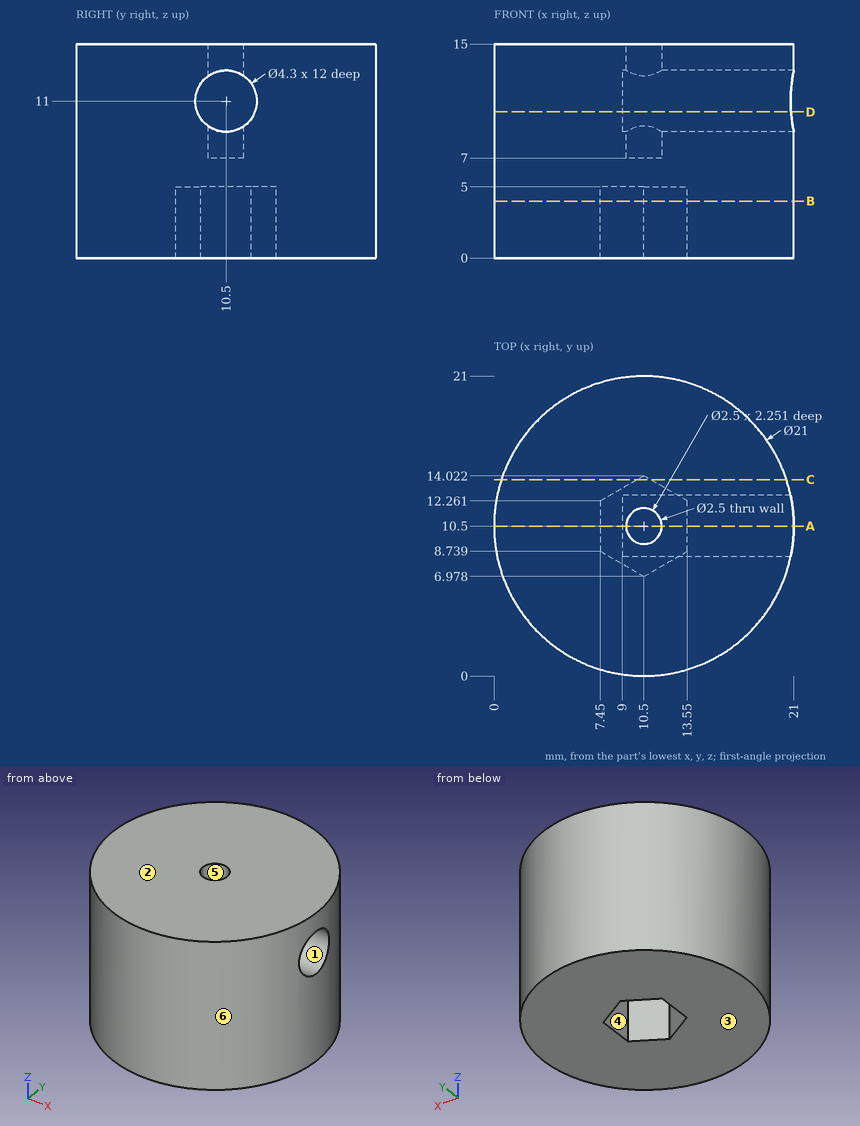
Geometry check sheet. Reference: drawing and pictorial views, mm from the part's lowest x, y, z. A direction names the side the tool comes from. Give positions to 0.01 mm unless a question says otherwise; leave off trailing zeros. Order: outer loops, then holes, each group sorted by start corner. A loop starts at its lowest first (then second) coordinate and runs counter-clockwise, first axis right, second up. Notation, with made-up numbers: M 50,89 L 70,89 A27 ccw 70,125 Z; hole C 12.25,19 d9. An arc over 180 degrees is marked long. Answer in a Markdown table with one row per item. Add a question column.
Q1. Sectioned sample at B-B, the plane z = 4. Record the boundary of the cut face in (x, y), and give its area (3 significant figures).
Q2. Thickness scan on L1, parallel to Y at x = 10.5, z = 7.8; L2, parallel to Y at x = 12.5, z = 10; L3, parallel to X at y = 19.25, z = 6.5 (1 decimal). Record the ranges inside material, lowest first.
Q3. Sectioned sample at C-C, the plane y = 13.75. Record the boundary of the cut face in (x, z), and give its area (3 significant figures).
Q4. Sectioned sample at D-D, the plane z = 10.25. Record the boundary of the cut face in (x, y) (1 decimal), and give its area (3 significant figures).
Q5. Release check for a two-part mould opening along Z. For the marked faces 1, 2 and 3 record: released by +Z, released by -Z, zero draft, split by the parting line, or undercut.
Q6. Sectioned sample at A-A, the plane y = 10.5. Record the boundary of the cut face in (x, z), and give its area (3 significant figures).
Q7. Gauge pin test, flat ends, axial feed: pin 1 Ø1 at (x, z) = (6, 9) entering from +Y; pin 2 Ø1 at (x, z) = (8.5, 9) entering from -Y; pin 3 Ø4 at (x, z) = (15, 7) entering from +Y. Record the tip position at first contact, or that the pin passes through.
Q8. Access from +Z, -Z, +X, -X, +Y, -Y to the whole of each face (thin tool, end or side, straight path). Record for the marked faces 4, 5 and 6.
Verdict:
| question | item | result |
|---|---|---|
| 1 | outline | C 10.5,10.5 d21; hole M 7.45,8.74 L 10.5,6.98 L 13.55,8.74 L 13.55,12.26 L 10.5,14.02 L 7.45,12.26 Z |
| 1 | area | 314 mm² |
| 2 | L1 | 0 to 9.25, 11.75 to 21 |
| 2 | L2 | 0.19 to 8.6, 12.4 to 20.81 |
| 2 | L3 | 4.7 to 16.3 |
| 3 | outline | M 0.52,0 L 10.03,0 L 10.03,5 L 10.97,5 L 10.97,0 L 20.48,0 L 20.48,15 L 0.52,15 Z |
| 3 | area | 295 mm² |
| 4 | outline | M 9,8.5 L 9,12.5 L 20.8,12.5 A10.5 ccw long 20.8,8.5 Z |
| 4 | area | 298 mm² |
| 5 | face 1 | undercut |
| 5 | face 2 | released by +Z |
| 5 | face 3 | released by -Z |
| 6 | outline | M 0,0 L 7.45,0 L 7.45,5 L 13.55,5 L 13.55,0 L 21,0 L 21,8.85 L 11.75,8.85 L 11.75,7 L 9.25,7 L 9.25,8.85 L 9,8.85 L 9,13.15 L 9.25,13.15 L 9.25,15 L 0,15 Z; M 11.75,13.15 L 21,13.15 L 21,15 L 11.75,15 Z |
| 6 | area | 224 mm² |
| 7 | pin 1 | y = 20.21 |
| 7 | pin 2 | y = 0.11 |
| 7 | pin 3 | y = 20.7 |
| 8 | face 4 | -Z |
| 8 | face 5 | +Z |
| 8 | face 6 | +Z, -Z |
